Can you work these out from the model? Positions are in its coordinate system, mm. A direction names the side the tool comes from. Give positions to 0.01 mm unless a question says otherwise; leave off trailing zeros. Order: outer loops, then holes, each group sorted by start corner. A loop starts at its lowest first (then second) coordinate and runs counter-clockwise, first axis right, second up. Notation, with made-up numbers: M 82.25,17 L 115.25,17 A16 ccw 115.25,35 Z; hole C 85,83 d2. An arc over 180 degrees is marked long. Use one line per item in the form item = value. Start each with the question number.
1. I want a section at A-A, the plane y = 0. List the corners of the cut face in (x, z) for me, and give its area (3 significant figures).
2. Will these pins go through, and if not, where does the flat tip stop? P1, Ø1.5, axis at x = 2.5, z = 108, coming from the +Y side; P2, Ø8, axis at x = 5.5, y = 11.5, coming from the +Z side; P3, Ø12, axis at x = 11, y = 5.5, coming from the +Z side; P4, Ø2, axis at x = -6.5, z = 102, coming from the +Y side (3 decimals).
3. For faces 1 (the face through (0, 0, -50)), 2 (the face through (4.006, 1.262, -31.872)), which set-ups out of +Z, -Z, +X, -X, +Y, -Y let a thin tool reach every point of the face, with its end or its side?
4. I want a section at D-D, the plane y = 12.5. List the corners of the cut face in (x, z) for me, and give its area (3 significant figures).
5. I want a section at C-C, the plane z = 23. List the corners of the cut face in (x, y) for me.
6. I need wall thicknesses on L1, parallel to Z at x = -8, y = 5.5; L2, parallel to X at y = -0.25, z = 3; L3, parallel to Y at x = 3.25, z = 28. Which ranges of each line are inside material? Lowest first, please.
```python
from build123d import *

# Parameters (mm, degrees)
CUT_EXTRUDE1_DEPTH      = 26.720954492
CUT_EXTRUDE1_DEPTH_BACK = 26.720954492
SKETCH2_R               = 4.2
SKETCH3_R               = 4.2
BOSS_EXTRUDE1_DEPTH     = 100
CUT_EXTRUDE2_START      = -50
SKETCH4_R               = 4.2
CUT_EXTRUDE2_DEPTH      = 50
BOSS_EXTRUDE2_START     = 50
SKETCH5_R               = 4.2
BOSS_EXTRUDE2_DEPTH     = 50


with BuildPart() as part:
    # Sketch1 → Revolve1 (revolve)
    with BuildSketch(Plane.XY):
        with BuildLine():
            Line((0, 14.85), (0, -14.85))
            ThreePointArc((0, -14.85), (14.85, 0), (0, 14.85))
        make_face()
    revolve(axis=Axis((0, 14.85, 0), (0, -1, 0)))

    # Sketch2 → Cut-Extrude1 (cut, two sides: drawn at the far end of the back side and taken through both)
    with BuildSketch(Plane.XY.offset(-CUT_EXTRUDE1_DEPTH_BACK)):
        with Locations(Location((0, 0, 0), (0, 0, 180))):
            Circle(SKETCH2_R)
    extrude(amount=CUT_EXTRUDE1_DEPTH + CUT_EXTRUDE1_DEPTH_BACK, mode=Mode.SUBTRACT)

    # Sketch3 → Boss-Extrude1 (add, symmetric)
    with BuildSketch(Plane.XY):
        Circle(SKETCH3_R)
    extrude(amount=BOSS_EXTRUDE1_DEPTH, both=True)

    # Sketch4 → Cut-Extrude2 (cut)
    with BuildSketch(Plane(origin=(0, 0, -100), x_dir=(-1, 0, 0), z_dir=(0, 0, -1)).offset(CUT_EXTRUDE2_START)):
        Circle(SKETCH4_R)
    extrude(amount=CUT_EXTRUDE2_DEPTH, mode=Mode.SUBTRACT)

    # Sketch5 → Boss-Extrude2 (add)
    with BuildSketch(Plane.XY.offset(100).offset(BOSS_EXTRUDE2_START)):
        with Locations(Location((0, 0, 0), (0, 0, 180))):
            Circle(SKETCH5_R)
    extrude(amount=-BOSS_EXTRUDE2_DEPTH)


solid = part.part
```
Check result:
q1.outline = M -4.2,-50 L 4.2,-50 L 4.2,-14.24 A14.85 ccw 4.2,14.24 L 4.2,150 L -4.2,150 L -4.2,14.24 A14.85 ccw -4.2,-14.24 Z
q1.area = 2,130 mm2
q2.P1 = 3.82
q2.P2 = 12
q2.P3 = 13.45
q2.P4 = through
q3.face_1 = -Z, +X, -X, +Y, -Y
q3.face_2 = -Z
q4.outline = C 0,0 d16.03
q4.area = 202 mm2
q5.outline = C 0,0 d8.4
q6.L1 = -11.24 to 11.24
q6.L2 = -14.54 to 14.54
q6.L3 = -2.66 to 2.66
